Build history of the part. All positions in model axes, mm. Face numbers are marked on the shaded views. A direction names the side the tool comes from. Give positions to 0.01 mm unless a question says otherwise; leave off trailing zeros. Write each loop counter-clockwise with the first axis right and the second up, starting at its lowest first coordinate (ties: lowest second). Pieces come first, ordered by that corner, then holes. Notation, with made-up numbers: M 73,-28.5 L 115,-28.5 A31 cw 115,8.5 Z; hole C 1,30 d9. An arc over 180 degrees is marked long. Return JSON: item names as keys, results as strings. Group by question number.
Q1. Band-saw the part on A-A, the plane z = 4. Give the cut face in (x, y).
Q2. Tool access for the marked faces 1, 2, 3 and 4: list every direction of +Z, -Z, +X, -X, +Y, -Y with a clear straight run to the whole face (end or side of a thin tool).
Q3. Flat gauge pins, fed straight in: pin 1 Ø2.5 at (x, y) = (3.75, -3.9) entering from -Z; pin 2 Ø2 at (x, y) = (6, -5.5) entering from +Z; pin 3 Ø1.6 at (x, y) = (3.5, -3.5) entering from +Z. Where does each tip first touch, or does it go through?
Q4. Pull direction X, two halves, no side cores. Call the marked faces 5, 6 and 7: +X half, -X half, draft (parallel to the pull), parting line (faces both ways), or undercut.
Q5. Band-saw the part on D-D, the plane x = 10. Give the cut face in (y, z), then the cut area to 3 significant figures.
Q6. Wall check: probe 1 along Z at (x, y) = (8.75, -6.25); probe 2 along Y at (x, z) = (5, 1); probe 3 along X at (y, z) = (-2, 1.25). Give the ranges that are in metal, low to high.
Q7. Band-saw the part on C-C, the plane x = 13.5. Give the cut face in (y, z), then the cut area to 3 significant figures.
Q8. Band-saw the part on B-B, the plane x = 8.25. Give the cut face in (y, z), then the cut area to 3 significant figures.
from build123d import *

# Parameters (mm, degrees)
F0_W     = 15.6
F0_H     = 9.6
F1_DEPTH = 7.8
F2_R     = 2.4
F2_R_2   = 1.6
F3_DEPTH = 1.7
F5_DEPTH = 2


# Not quite as in the source:
# - a feature names something its author has since deleted; it is built from what else it names


with BuildPart() as f1:
    # F0 (on Front) → F1 (new body)
    with BuildSketch(Plane.XZ):
        with Locations((7.5497636572, 4.7150965011)):
            Rectangle(F0_W, F0_H)
        with BuildLine():
            Line((10.5497636572, 6.6150965011), (10.5497636572, 5.6150965011))
            Line((10.5497636572, 5.6150965011), (10.5497636572, 4.6150965011))
            Line((10.5497636572, 4.6150965011), (10.3781907819, 4.6150965011))
            ThreePointArc((10.3781907819, 4.6150965011), (9.6710840007, 3.4937761575), (8.5497636572, 2.7866693764))
            Line((8.5497636572, 2.7866693764), (8.5497636572, 2.6150965011))
            Line((8.5497636572, 2.6150965011), (7.5497636572, 2.6150965011))
            Line((7.5497636572, 2.6150965011), (6.5497636572, 2.6150965011))
            Line((6.5497636572, 2.6150965011), (6.5497636572, 2.7866693764))
            ThreePointArc((6.5497636572, 2.7866693764), (5.4284433136, 3.4937761575), (4.7213365324, 4.6150965011))
            Line((4.7213365324, 4.6150965011), (4.5497636572, 4.6150965011))
            Line((4.5497636572, 4.6150965011), (4.5497636572, 5.6150965067))
            Line((4.5497636572, 5.6150965067), (4.5497636572, 6.6150965011))
            Line((4.5497636572, 6.6150965011), (4.7213365324, 6.6150965011))
            ThreePointArc((4.7213365324, 6.6150965011), (5.4284433136, 7.7364168447), (6.5497636572, 8.4435236258))
            Line((6.5497636572, 8.4435236258), (6.5497636572, 8.6150965011))
            Line((6.5497636572, 8.6150965011), (7.5497636572, 8.6150965011))
            Line((7.5497636572, 8.6150965011), (8.5497636572, 8.6150965011))
            Line((8.5497636572, 8.6150965011), (8.5497636572, 8.4435236258))
            ThreePointArc((8.5497636572, 8.4435236258), (9.6710840007, 7.7364168447), (10.3781907819, 6.6150965011))
            Line((10.3781907819, 6.6150965011), (10.5497636572, 6.6150965011))
        make_face(mode=Mode.SUBTRACT)
        with BuildLine():
            ThreePointArc((8.5497636572, 2.7866693764), (9.6710840007, 3.4937761575), (10.3781907819, 4.6150965011))
            Line((10.3781907819, 4.6150965011), (8.5497636572, 4.6150965011))
            Line((8.5497636572, 4.6150965011), (8.5497636572, 2.7866693764))
        make_face()
        with BuildLine():
            Line((8.5497636572, 6.6150965011), (10.3781907819, 6.6150965011))
            ThreePointArc((10.3781907819, 6.6150965011), (9.6710840007, 7.7364168447), (8.5497636572, 8.4435236258))
            Line((8.5497636572, 8.4435236258), (8.5497636572, 6.6150965011))
        make_face()
        with BuildLine():
            Line((4.7213365324, 6.6150965011), (6.5497636572, 6.6150965011))
            Line((6.5497636572, 6.6150965011), (6.5497636572, 8.4435236258))
            ThreePointArc((6.5497636572, 8.4435236258), (5.4284433136, 7.7364168447), (4.7213365324, 6.6150965011))
        make_face()
        with BuildLine():
            Line((6.5497636572, 2.7866693764), (6.5497636572, 4.6150965011))
            Line((6.5497636572, 4.6150965011), (4.7213365324, 4.6150965011))
            ThreePointArc((4.7213365324, 4.6150965011), (5.4284433136, 3.4937761575), (6.5497636572, 2.7866693764))
        make_face()
        with BuildLine():
            Line((10.5497636572, 4.6150965011), (10.5497636572, 5.6150965011))
            ThreePointArc((10.5497636572, 5.6150965011), (10.5065593361, 5.1077905649), (10.3781907819, 4.6150965011))
            Line((10.3781907819, 4.6150965011), (10.5497636572, 4.6150965011))
        make_face()
        with BuildLine():
            ThreePointArc((10.3781907819, 6.6150965011), (10.5065593361, 6.1224024373), (10.5497636572, 5.6150965011))
            Line((10.5497636572, 5.6150965011), (10.5497636572, 6.6150965011))
            Line((10.5497636572, 6.6150965011), (10.3781907819, 6.6150965011))
        make_face()
        with BuildLine():
            ThreePointArc((7.5497636572, 8.6150965011), (8.0570695933, 8.5718921801), (8.5497636572, 8.4435236258))
            Line((8.5497636572, 8.4435236258), (8.5497636572, 8.6150965011))
            Line((8.5497636572, 8.6150965011), (7.5497636572, 8.6150965011))
        make_face()
        with BuildLine():
            ThreePointArc((6.5497636572, 8.4435236258), (7.042457721, 8.5718921801), (7.5497636572, 8.6150965011))
            Line((7.5497636572, 8.6150965011), (6.5497636572, 8.6150965011))
            Line((6.5497636572, 8.6150965011), (6.5497636572, 8.4435236258))
        make_face()
        with BuildLine():
            ThreePointArc((4.5497636572, 5.6150965067), (4.5929679787, 6.12240244), (4.7213365324, 6.6150965011))
            Line((4.7213365324, 6.6150965011), (4.5497636572, 6.6150965011))
            Line((4.5497636572, 6.6150965011), (4.5497636572, 5.6150965067))
        make_face()
        with BuildLine():
            Line((4.5497636572, 4.6150965011), (4.7213365324, 4.6150965011))
            ThreePointArc((4.7213365324, 4.6150965011), (4.5929679777, 5.1077905677), (4.5497636572, 5.6150965067))
            Line((4.5497636572, 5.6150965067), (4.5497636572, 4.6150965011))
        make_face()
        with BuildLine():
            Line((6.5497636572, 2.6150965011), (7.5497636572, 2.6150965011))
            ThreePointArc((7.5497636572, 2.6150965011), (7.042457721, 2.6583008221), (6.5497636572, 2.7866693764))
            Line((6.5497636572, 2.7866693764), (6.5497636572, 2.6150965011))
        make_face()
        with BuildLine():
            Line((8.5497636572, 2.6150965011), (8.5497636572, 2.7866693764))
            ThreePointArc((8.5497636572, 2.7866693764), (8.0570695933, 2.6583008221), (7.5497636572, 2.6150965011))
            Line((7.5497636572, 2.6150965011), (8.5497636572, 2.6150965011))
        make_face()
    extrude(amount=F1_DEPTH)

    # F2 (on face) → F3 (join)
    with BuildSketch(Plane.XY.offset(9.5150965011)):
        with Locations((3.7497636572, -3.9)):
            Circle(F2_R)
        with Locations((3.7497636572, -3.9)):
            Circle(F2_R_2, mode=Mode.SUBTRACT)
        with Locations((11.3497636572, -3.9)):
            Circle(F2_R)
        with Locations((11.3497636572, -3.9)):
            Circle(F2_R_2, mode=Mode.SUBTRACT)
    extrude(amount=F3_DEPTH)

    # F4 (on face) → F5 (cut)
    with BuildSketch(Plane(origin=(0, 0, -0.0849034989), x_dir=(1, 0, 0), z_dir=(0, 0, -1))):
        Polygon((1.3497636572, 6.2), (1.3497636572, 3.9), (1.3497636572, 1.6), (7.5497636572, 1.6), (13.7497636572, 1.6), (13.7497636572, 3.9), (13.7497636572, 6.2), (7.5497636572, 6.2), align=None)
    extrude(amount=-F5_DEPTH, mode=Mode.SUBTRACT)


solid = f1.part
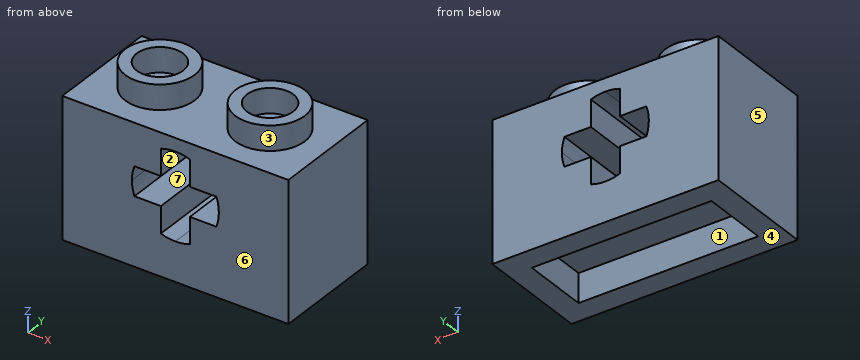
From the geometry:
{
 "1": {"outline": "M -0.25,-7.8 L 6.55,-7.8 L 6.55,0 L -0.25,0 Z; M 8.55,-7.8 L 15.35,-7.8 L 15.35,0 L 8.55,0 Z"},
 "2": {"face 1": "-Z", "face 2": "+Y, -Y", "face 3": "+Z", "face 4": "-Z, +X, -X, +Y, -Y"},
 "3": {"pin 1": "stops at z = 1.92", "pin 2": "stops at z = 11.22", "pin 3": "stops at z = 9.52"},
 "4": {"face 5": "-X half", "face 6": "draft", "face 7": "undercut"},
 "5": {"outline": "M -7.8,-0.08 L -6.2,-0.08 L -6.2,1.92 L -1.6,1.92 L -1.6,-0.08 L 0,-0.08 L 0,4.62 L -7.8,4.62 Z; M -7.8,6.62 L 0,6.62 L 0,9.52 L -1.92,9.52 L -1.92,11.22 L -3.04,11.22 L -3.04,9.52 L -4.76,9.52 L -4.76,11.22 L -5.88,11.22 L -5.88,9.52 L -7.8,9.52 Z", "area": "53.9 mm^2"},
 "6": {"probe 1": "z = -0.08 to 4.62, 6.62 to 9.52", "probe 2": "y = -7.8 to -6.2, -1.6 to 0", "probe 3": "x = -0.25 to 1.35, 13.75 to 15.35"},
 "7": {"outline": "M -7.8,-0.08 L -6.2,-0.08 L -6.2,1.92 L -1.6,1.92 L -1.6,-0.08 L 0,-0.08 L 0,9.52 L -2.83,9.52 L -2.83,11.22 L -4.97,11.22 L -4.97,9.52 L -7.8,9.52 Z", "area": "69.3 mm^2"},
 "8": {"outline": "M -7.8,-0.08 L -6.2,-0.08 L -6.2,1.92 L -1.6,1.92 L -1.6,-0.08 L 0,-0.08 L 0,2.7 L -7.8,2.7 Z; M -7.8,8.53 L 0,8.53 L 0,9.52 L -7.8,9.52 Z", "area": "20.2 mm^2"}
}
